The listing builds one solid part. Answer for the finished solid, in the listing's coordinates (mm). Face numbers are marked on the shaded views. A direction names the side the tool comes from. Coordinates: 2 decimals unless noted, no trailing zeros. Loops run counter-clockwise (first coordinate to the right, second up) from the corner with the lowest first, then second, coordinate; pieces in that order, holes last. Notation, with made-up numbers: M -30.75,-19.5 L -18.75,-19.5 A12 ccw -18.75,-5.5 Z; hole C -14.75,-34 d2. An arc over 180 degrees is marked long. Answer in a Markdown table with one row per item. Add a question column.
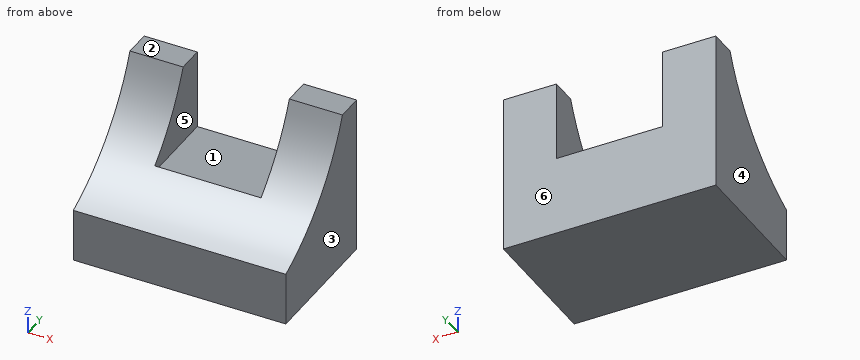
from build123d import *

# Parameters (mm, degrees)
F0_W     = 31.75
F0_H     = 38.1
F1_DEPTH = 50.8
F3_DEPTH = 50.8
F4_W     = 25.4
F4_H     = 19.05
F5_DEPTH = 19.05


with BuildPart() as f1:
    # F0 (on Right) → F1 (new body)
    with BuildSketch(Plane.YZ):
        with Locations((-10.51228, 19.05)):
            Rectangle(F0_W, F0_H)
    extrude(amount=-F1_DEPTH)

    # F2 (on face) → F3 (cut)
    with BuildSketch(Plane.YZ):
        with BuildLine():
            Line((-26.38728, 38.1), (-26.38728, 12.7))
            ThreePointArc((-26.38728, 12.7), (-11.141967, 22.854688), (-0.98728, 38.1))
            Line((-0.98728, 38.1), (-26.38728, 38.1))
        make_face()
    extrude(amount=-F3_DEPTH, mode=Mode.SUBTRACT)

    # F4 (on face) → F5 (cut)
    with BuildSketch(Plane(origin=(0, 5.36272, 0), x_dir=(-1, 0, 0), z_dir=(0, 1, 0))):
        with Locations((25.4, 28.575)):
            Rectangle(F4_W, F4_H)
    extrude(amount=-F5_DEPTH, mode=Mode.SUBTRACT)


solid = f1.part
(1) This flat-tipped pin is pushed along its axis until it touches: pin 1 (2 mm diameter, centred on x = -35.5, z = 21, fed in from +Y). Where does it stop, or does it pass through?
(2) A cutting plane is placed at A-A (z = 25.5). Give the vertices of the cut face in (x, y).
(3) A cutting plane is placed at C-C (y = -12). Give the vertices of the cut face in (x, z), plus the area to 3 significant figures.
(4) A cutting plane is placed at D-D (z = 33.5). Give the vertices of the cut face in (x, y).
(5) Straight lines are drawn through the part: line 1 (X direction, y = -6.5, z = 26); line 2 (Z direction, x = -32.5, y = 2); line 3 (Y direction, x = -38.5, z = 29.5). For each, find the intervals that lie inside material, in ascending order.
(6) For the marked faces 1 and 2, determine the directions among +Z, -Z, +X, -X, +Y, -Y from which every point of the face is accessible in a straight line to the end or side of a thin tool.
(7) The mould has two halves that part along X. Classify the marked faces 3, 4, 5 and 6: released by +X, released by -X, zero draft, split by the parting line, or undercut.
(8) A cutting plane is placed at B-B (x = -15). Give the vertices of the cut face in (y, z), plus the area to 3 significant figures.
Solved:
| question | item | result |
|---|---|---|
| 1 | pin 1 | stops at y = -13.69 |
| 2 | outline | M -50.8,-8.69 L -38.1,-8.69 L -38.1,5.36 L -50.8,5.36 Z; M -12.7,-8.69 L 0,-8.69 L 0,5.36 L -12.7,5.36 Z |
| 3 | outline | M -50.8,0 L 0,0 L 0,22.02 L -12.7,22.02 L -12.7,19.05 L -38.1,19.05 L -38.1,22.02 L -50.8,22.02 Z |
| 3 | area | 1,040 mm² |
| 4 | outline | M -50.8,-3.18 L -38.1,-3.18 L -38.1,5.36 L -50.8,5.36 Z; M -12.7,-3.18 L 0,-3.18 L 0,5.36 L -12.7,5.36 Z |
| 5 | line 1 | x = -50.8 to -38.1, -12.7 to 0 |
| 5 | line 2 | z = 0 to 19.05 |
| 5 | line 3 | y = -5.63 to 5.36 |
| 6 | face 1 | +Z, +Y |
| 6 | face 2 | +Z, +X, -X, +Y, -Y |
| 7 | face 3 | released by +X |
| 7 | face 4 | released by -X |
| 7 | face 5 | undercut |
| 7 | face 6 | zero draft |
| 8 | outline | M -26.39,0 L 5.36,0 L 5.36,19.05 L -13.69,19.05 L -13.69,20.49 A46.61 cw -26.39,12.7 Z |
| 8 | area | 568 mm² |
